Can you work these out from the model? Positions are in its coordinate system, mm. A direction names the side the tool comes from. Give positions to 0.01 mm unless a question says otherwise; leave off trailing zeros. Loops run counter-clockwise (first coordinate to the right, second up) from the corner with the lowest first, then second, coordinate; pieces in that order, holes last.
from build123d import *

# Parameters (mm, degrees)
SKETCH051_R             = 1.35
PAD051_DEPTH            = 9.7
SKETCH052_W             = 2.9
SKETCH052_H             = 4.1
PAD052_DEPTH            = 3
SKETCH053_W             = 0.8
SKETCH053_H             = 6.4
PAD053_DEPTH            = 10
SKETCH054_W             = 0.8
SKETCH054_H             = 6.4
PAD054_DEPTH            = 3
SKETCH055_W             = 0.8
SKETCH055_H             = 6.4
PAD055_DEPTH            = 9.3
FILLET007_R             = 1.2
BODY011_PLACEMENT_ANGLE = 90


with BuildPart() as part:
    # Sketch051 → Pad051 (new body)
    with BuildSketch(Plane.XY):
        with BuildLine():
            ThreePointArc((-12.25, 8), (-13.487437, 7.487437), (-14, 6.25))
            Line((-14, -6.25), (-14, 6.25))
            ThreePointArc((-14, -6.25), (-13.487437, -7.487437), (-12.25, -8))
            Line((12.25, -8), (-12.25, -8))
            ThreePointArc((12.25, -8), (13.487437, -7.487437), (14, -6.25))
            Line((14, 6.25), (14, -6.25))
            ThreePointArc((14, 6.25), (13.487437, 7.487437), (12.25, 8))
            Line((-12.25, 8), (12.25, 8))
        make_face()
        with Locations((10.877931, -4.825)):
            Circle(SKETCH051_R, mode=Mode.SUBTRACT)
        with Locations((-10.877931, 4.825)):
            Circle(SKETCH051_R, mode=Mode.SUBTRACT)
    extrude(amount=PAD051_DEPTH)

    # Sketch052 (on Face8 of Pad051) → Pad052 (join)
    with BuildSketch(Plane(origin=(0, 8, 0), x_dir=(-1, 0, 0), z_dir=(0, 1, 0))):
        with Locations((-9.45, 4.85)):
            Rectangle(SKETCH052_W, SKETCH052_H)
    extrude(amount=PAD052_DEPTH)

    # Sketch053 (on Face3 of Pad052) → Pad053 (join)
    with BuildSketch(Plane(origin=(-14, 0, 0), x_dir=(0, -1, 0), z_dir=(-1, 0, 0))):
        with Locations((4.3, 4.85)):
            Rectangle(SKETCH053_W, SKETCH053_H)
    extrude(amount=PAD053_DEPTH)

    # Sketch054 (on Face16 of Pad053) → Pad054 (join)
    with BuildSketch(Plane.XZ.offset(8)):
        with Locations((-0.9, 4.85)):
            Rectangle(SKETCH054_W, SKETCH054_H)
    extrude(amount=PAD054_DEPTH)

    # Sketch055 (on Face23 of Pad054) → Pad055 (join)
    with BuildSketch(Plane(origin=(-1.3, 0, 0), x_dir=(0, -1, 0), z_dir=(-1, 0, 0))):
        with Locations((10.6, 4.85)):
            Rectangle(SKETCH055_W, SKETCH055_H)
    extrude(amount=PAD055_DEPTH)

    # Fillet007
    fillet007_edges = [part.edges().sort_by_distance(p)[0] for p in [
        (10.9, 11, 4.85),
        (8, 11, 4.85),
    ]]
    fillet(fillet007_edges, radius=FILLET007_R)


with BuildPart() as part_1:
    # Body011 placement: moved
    add(part.part.moved(Location((192.8, 0, -97))).rotate(Axis((192.8, 0, -97), (0, 1, 0)), BODY011_PLACEMENT_ANGLE))


solid = part_1.part
(1) Which directions (+Z, -Z, +X, -X, +Y, -Y) give clear straight access to the entire face, cutting with the end or side of a thin tool? Please do faces 4 (the flat face through (200.85, -10.5, -92.6)), 5 (the flat face through (199.7, 9, -106)), 6 (the flat face through (195.6, 9, -106)), 7 (the flat face through (198, -4.7, -78)), 8 (the flat face through (194.45, -4.3, -78.1)).
Returned:
face 4: +Z, -Z, +X, -Y
face 5: +Z, -Z, +X, +Y
face 6: +Z, -Z, -X, +Y
face 7: +Z, +X, -X, -Y
face 8: +Z, -X, +Y, -Y
(2) Suppose I cut it at B-B on z = -98. List the corners of the cut face in (x, y) for me, plus the area to 3 significant figures.
Returned:
outline: (192.8, -8) - (202.5, -8) - (202.5, 8) - (192.8, 8) - close
area: 155 mm2
(3) Thinking about a two-plate mould opening in Y: for faces 1 (the flat face through (198, 9, -107.9)), 2 (the flat face through (198, -3.9, -78)), 3 (the flat face through (198, -9, -95.7)), which applies, pulls with the +Y half, pulls with the -Y half, needs draft (parallel to the pull), parting line crosses it, or undercut?
Returned:
face 1: needs draft
face 2: pulls with the +Y half
face 3: undercut
(4) Please list where these lines run through material, in increasing order: probe 1 along Y at (x, z) = (198, -108); probe 2 along Y at (x, z) = (200.75, -86); probe 3 along Z at (x, y) = (196, -1.5).
Returned:
probe 1: y = -8 to -6.17, -3.48 to 8
probe 2: y = -8 to 3.48, 6.17 to 8
probe 3: z = -111 to -83
(5) Will these pins go through, and if not, where does the flat tip stop? P1, Ø5, axis at x = 194.5, z = -79, coming from the +Y side; P2, Ø3, axis at x = 197, z = -92, coming from the +Y side; P3, Ø0.9, axis at y = -4.5, z = -76, coming from the +X side.
Returned:
P1: stops at y = -3.9
P2: stops at y = 8
P3: stops at x = 200.85
(6) Suppose I cut it at A-A on y = 8.5. List the corners of the cut face in (x, z) for me.
Returned:
outline: (195.6, -107.9) - (199.7, -107.9) - (199.7, -105) - (195.6, -105) - close
(7) Suppose I cut it at C-C on x = 199. List the corners of the cut face in (y, z) for me (3 decimals), plus the area to 3 significant figures.
Returned:
outline: (-11, -96.5) - (-8, -96.5) - (-8, -109.25) arc R1.75 ccw to (-6.25, -111) - (6.25, -111) arc R1.75 ccw to (8, -109.25) - (8, -107.9) - (9.8, -107.9) arc R1.2 ccw to (11, -106.7) - (11, -106.2) arc R1.2 ccw to (9.8, -105) - (8, -105) - (8, -84.75) arc R1.75 ccw to (6.25, -83) - (-3.9, -83) - (-3.9, -73) - (-4.7, -73) - (-4.7, -83) - (-6.25, -83) arc R1.75 ccw to (-8, -84.75) - (-8, -95.7) - (-10.2, -95.7) - (-10.2, -86.4) - (-11, -86.4) - close; hole circle Ø2.7 at (-4.825, -107.878); hole circle Ø2.7 at (4.825, -86.122)
area: 460 mm2
